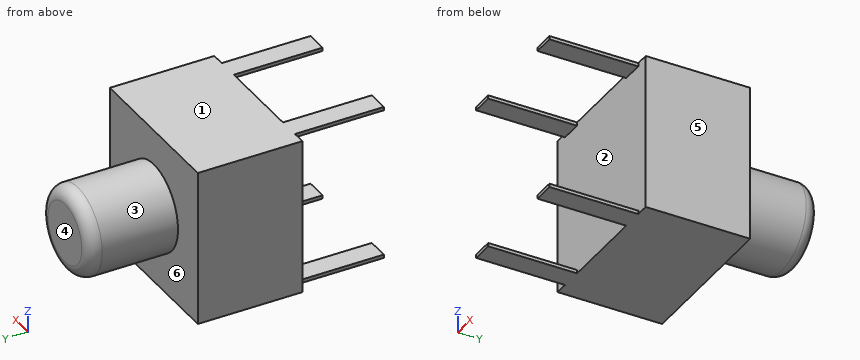
```python
from build123d import *

# Parameters (mm, degrees)
ESQUISSE1_W                                = 6
ESQUISSE1_H                                = 6
BOSS_EXTRU_1_DEPTH                         = 4
ESQUISSE2_R                                = 1.65
BOSS_EXTRU_2_DEPTH                         = 3.4
CONG_1_R                                   = 0.5
ESQUISSE3_W                                = 0.819968842
ESQUISSE3_H                                = 0.132597198
BOSS_EXTRU_3_DEPTH                         = 3.4
SYM_TRIE1_AT_THE_SECOND_PLANE_COPY_1_SKE_W = 0.819968842
SYM_TRIE1_AT_THE_SECOND_PLANE_COPY_1_SKE_H = 0.132597198
SYM_TRIE1_AT_THE_SECOND_PLANE_COPY_1_DEPTH = 3.4


with BuildPart() as part:
    # Esquisse1 → Boss.-Extru.1 (new body)
    with BuildSketch(Plane(origin=(0, 0, 0), x_dir=(1, 0, 0), z_dir=(0, 1, 0))):
        Rectangle(ESQUISSE1_W, ESQUISSE1_H)
    extrude(amount=BOSS_EXTRU_1_DEPTH)

    # Esquisse2 → Boss.-Extru.2 (add)
    with BuildSketch(Plane(origin=(0, 4, 0), x_dir=(1, 0, 0), z_dir=(0, 1, 0))):
        with Locations(Location((0, 0, 0), (0, 0, 270))):
            Circle(ESQUISSE2_R)
    extrude(amount=BOSS_EXTRU_2_DEPTH)

    # Cong_1
    cong_1_edges = [part.edges().sort_by_distance(p)[0] for p in [
        (0, 7.4, -1.65),
    ]]
    fillet(cong_1_edges, radius=CONG_1_R)

    # Esquisse3 → Boss.-Extru.3 (add)
    with BuildSketch(Plane.XZ):
        with Locations((-2.087621823, -2.933701401)):
            Rectangle(ESQUISSE3_W, ESQUISSE3_H)
    boss_extru_3 = extrude(amount=BOSS_EXTRU_3_DEPTH)

    # Sym_trie1: Boss.-Extru.3 across plane
    add(boss_extru_3.mirror(Plane(origin=(0, 0, 0), x_dir=(0, 0, 1), z_dir=(1, 0, 0))))

    # Sym_trie1 at the second plane: Boss.-Extru.3 across plane
    add(boss_extru_3.mirror(Plane.XY))

    # Sym_trie1 at the second plane copy 1 ske → Sym_trie1 at the second plane copy 1 (add)
    with BuildSketch(Plane(origin=(0, 0, 0), x_dir=(-1, 0, 0), z_dir=(0, -1, 0))):
        with Locations((-2.087621823, -2.933701401)):
            Rectangle(SYM_TRIE1_AT_THE_SECOND_PLANE_COPY_1_SKE_W, SYM_TRIE1_AT_THE_SECOND_PLANE_COPY_1_SKE_H)
    extrude(amount=SYM_TRIE1_AT_THE_SECOND_PLANE_COPY_1_DEPTH)


solid = part.part
```
Design review of the part built by this model. Coordinates are the model's own, in mm. Face numbers are marked on the shaded views. A direction names the side the tool comes from. Coordinates: 2 decimals unless noted, no trailing zeros. Order: outer loops, then holes, each group sorted by start corner. A loop starts at its lowest first (then second) coordinate and runs counter-clockwise, first axis right, second up.
1) Take a section at D-D, the plane y = 5.75. Give the boundary of the cut face in (x, z), and give its area (3 significant figures).
2) Clearance check with a flat-ended pin moving along its axis: pin 1 (3 mm diameter, centred on x = 0, z = 0, fed in from -Y). State where the tip first meets the part, or that it passes through.
3) Wall thickness on line 1 along Y through (x, z) = (2.35, 1.65); line 2 along Y through (x, z) = (-0.15, -0.95); line 3 along X through (y, z) = (5, -1.5): over which ranges is each line inside the solid? List them lowest first.
4) Mouldability with a two-part tool opening along Z and no side actions: class the marked faces 1, 2, 3 and 4 as +Z half, -Z half, draft (parallel to the pull), parting line (faces both ways), or undercut.
5) Take a section at A-A, the plane y = -1.5. Give the boundary of the cut face in (x, z), and give its area (3 significant figures).
6) Take a section at B-B, the plane z = 0. Give the boundary of the cut face in (x, y), and give its area (3 significant figures).
7) Take a section at C-C, the plane x = 0. Give the boundary of the cut face in (y, z), and give its area (3 significant figures).
8) For the marked faces 5 and 6, list the 3-axis set-ups (+Z, -Z, +X, -X, +Y, -Y) from which the entire face can be reached by the end or side of a thin tool; tool diameter is ignored.
Returned:
1. outline: circle Ø3.3 at (0, 0)
1. area: 8.55 mm2
2. pin 1: stops at y = 0
3. line 1: y = 0 to 4
3. line 2: y = 0 to 7.4
3. line 3: x = -0.69 to 0.69
4. face 1: +Z half
4. face 2: undercut
4. face 3: parting line
4. face 4: draft
5. outline: (-2.5, -3) - (-1.68, -3) - (-1.68, -2.87) - (-2.5, -2.87) - close; (-2.5, 2.87) - (-1.68, 2.87) - (-1.68, 3) - (-2.5, 3) - close; (1.68, -3) - (2.5, -3) - (2.5, -2.87) - (1.68, -2.87) - close; (1.68, 2.87) - (2.5, 2.87) - (2.5, 3) - (1.68, 3) - close
5. area: 0.435 mm2
6. outline: (-3, 0) - (3, 0) - (3, 4) - (1.65, 4) - (1.65, 6.9) arc R0.5 ccw to (1.15, 7.4) - (-1.15, 7.4) arc R0.5 ccw to (-1.65, 6.9) - (-1.65, 4) - (-3, 4) - close
6. area: 35.1 mm2
7. outline: (0, -3) - (4, -3) - (4, -1.65) - (6.9, -1.65) arc R0.5 ccw to (7.4, -1.15) - (7.4, 1.15) arc R0.5 ccw to (6.9, 1.65) - (4, 1.65) - (4, 3) - (0, 3) - close
7. area: 35.1 mm2
8. face 5: +Z, -Z, +X, +Y, -Y
8. face 6: +Y
